Check sheet for the modelled part. Datum: model origin and axes. Units: mm. Round coordinates to 2 decimals unless told otherwise and drop trailing zeros. Loops run counter-clockwise (first coordinate to the right, second up) from the corner with the lowest first, then second, coordinate; pieces in that order, holes last. Notation, with made-up numbers: (80.5, -31) - (86.5, -31) arc R22 cw to (86.5, -17) - close; hole circle Ø9 at (61, 43.25). An arc over 180 degrees is marked (long way). Put each result on its own line as item: value.
```python
from build123d import *

# Parameters (mm, degrees)
F0_W     = 177.8
F0_H     = 127
F1_DEPTH = 127
F2_R     = 25.4


with BuildPart() as f1:
    # F0 (on Top) → F1 (new body)
    with BuildSketch(Plane.XY):
        with Locations((88.9, 63.5)):
            Rectangle(F0_W, F0_H)
    extrude(amount=F1_DEPTH)

    # F2
    f2_edges = [f1.edges().sort_by_distance(p)[0] for p in [
        (0, 63.5, 127),
        (88.9, 0, 127),
        (88.9, 127, 127),
        (177.8, 63.5, 127),
    ]]
    fillet(f2_edges, radius=F2_R)

    # F3: F1 across plane


with BuildPart() as f1_1:
    add(f1.part)
    add(f1.part.mirror(Plane.XZ))


solid = f1_1.part
```
Item 1: Go/stop test with a flat-tipped pin: pin 1 (12 mm diameter, centred on x = 95, z = 112, fed in from +Y). Record where the tip stops, or that it passes through.
Filled sheet:
pin 1: y = 126.62
Item 2: Section check B-B on y = -4. Enter the section's corners in (x, z), then the cut area to 3 significant figures.
Filled sheet:
outline: (0, 0) - (177.8, 0) - (177.8, 101.6) arc R25.4 ccw to (173.8, 115.28) - (4, 115.28) arc R25.4 ccw to (0, 101.6) - close
area: 20,500 mm²
Item 3: Section check A-A on x = 133.5. Enter the section's corners in (y, z), then the cut area to 3 significant figures.
Filled sheet:
outline: (-127, 0) - (127, 0) - (127, 101.6) arc R25.4 ccw to (101.6, 127) - (25.4, 127) arc R25.4 ccw to (0, 101.6) arc R25.4 ccw to (-25.4, 127) - (-101.6, 127) arc R25.4 ccw to (-127, 101.6) - close
area: 31,700 mm²
Item 4: Thickness scan on line 1 (Y direction, x = 24.5, z = 118.5); line 2 (Y direction, x = 154.5, z = 109.5); line 3 (X direction, y = 12, z = 102.5). Record the ranges inside material, lowest first. Write a range as from..to.
Filled sheet:
line 1: -120.56..-6.44, 6.44..120.56
line 2: -125.74..-1.26, 1.26..125.74
line 3: 0.02..177.78
